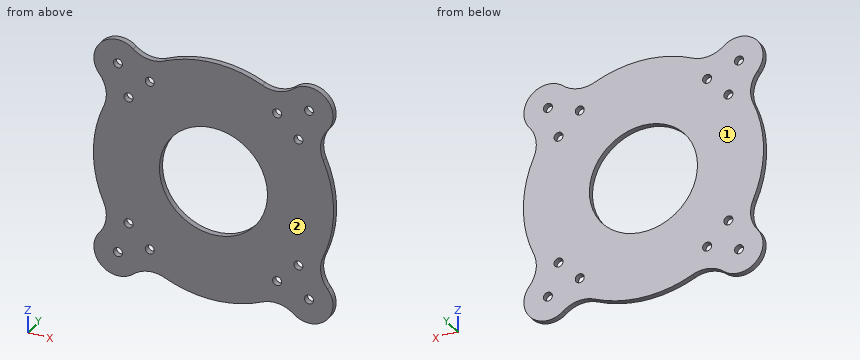
from build123d import *

# Parameters (mm, degrees)
SKETCH_1_R          = 40
SKETCH_1_R_2        = 18
EXTRUDE_1_DEPTH     = 2
EXTRUDE_2_DEPTH     = 2
FILLET_1_R          = 10
SKETCH_2_R          = 1.5
CUT_EXTRUDE_1_DEPTH = 57.603886937


with BuildPart() as part:
    # 草图1 → 凸台-拉伸1 (new body)
    with BuildSketch(Plane(origin=(0, 0, 0), x_dir=(1, 0, 0), z_dir=(0, 1, 0))):
        with Locations(Location((0, 0, 0), (0, 0, 270))):
            Circle(SKETCH_1_R)
        with Locations(Location((0, 0, 0), (0, 0, 270))):
            Circle(SKETCH_1_R_2, mode=Mode.SUBTRACT)
    extrude(amount=EXTRUDE_1_DEPTH)

    # 草图4 → 凸台-拉伸2 (add)
    with BuildSketch(Plane.XZ):
        with BuildLine():
            Line((19.091883092, 30.405591591), (26.162950904, 37.476659403))
            ThreePointArc((26.162950904, 37.476659403), (37.476659403, 37.476659403), (37.476659403, 26.162950904))
            Line((37.476659403, 26.162950904), (30.405591591, 19.091883092))
            ThreePointArc((30.405591591, 19.091883092), (19.091883092, 19.091883092), (19.091883092, 30.405591591))
        make_face()
        with BuildLine():
            Line((19.091883092, -30.405591591), (26.162950904, -37.476659403))
            ThreePointArc((26.162950904, -37.476659403), (37.476659403, -37.476659403), (37.476659403, -26.162950904))
            Line((37.476659403, -26.162950904), (30.405591591, -19.091883092))
            ThreePointArc((30.405591591, -19.091883092), (19.091883092, -19.091883092), (19.091883092, -30.405591591))
        make_face()
        with BuildLine():
            Line((-30.405591591, -19.091883092), (-37.476659403, -26.162950904))
            ThreePointArc((-37.476659403, -26.162950904), (-37.476659403, -37.476659403), (-26.162950904, -37.476659403))
            Line((-26.162950904, -37.476659403), (-19.091883092, -30.405591591))
            ThreePointArc((-19.091883092, -30.405591591), (-19.091883092, -19.091883092), (-30.405591591, -19.091883092))
        make_face()
        with BuildLine():
            Line((-19.091883092, 30.405591591), (-26.162950904, 37.476659403))
            ThreePointArc((-26.162950904, 37.476659403), (-37.476659403, 37.476659403), (-37.476659403, 26.162950904))
            Line((-37.476659403, 26.162950904), (-30.405591591, 19.091883092))
            ThreePointArc((-30.405591591, 19.091883092), (-19.091883092, 19.091883092), (-19.091883092, 30.405591591))
        make_face()
    extrude(amount=-EXTRUDE_2_DEPTH)

    # 圆角1
    fillet_1_edges = [part.edges().sort_by_distance(p)[0] for p in [
        (-22.055958672, 1, -33.369667171),
        (-33.369667171, 1, -22.055958672),
        (-33.369667171, 1, 22.055958672),
        (-22.055958672, 1, 33.369667171),
        (22.055958672, 1, 33.369667171),
        (33.369667171, 1, 22.055958672),
        (33.369667171, 1, -22.055958672),
        (22.055958672, 1, -33.369667171),
    ]]
    fillet(fillet_1_edges, radius=FILLET_1_R)

    # 草图2 → 切除-拉伸1 (cut, through all)
    with BuildSketch(Plane(origin=(0, 2, 0), x_dir=(1, 0, 0), z_dir=(0, 1, 0))):
        with Locations(Location((-21.213203436, -28.284271247, 0), (0, 0, 270))):
            Circle(SKETCH_2_R)
        with Locations(Location((-31.819805153, -31.819805153, 0), (0, 0, 270))):
            Circle(SKETCH_2_R)
        with Locations(Location((-28.284271247, -21.213203436, 0), (0, 0, 90))):
            Circle(SKETCH_2_R)
        with Locations(Location((-31.819805153, 31.819805153, 0), (0, 0, 270))):
            Circle(SKETCH_2_R)
        with Locations(Location((-21.213203436, 28.284271247, 0), (0, 0, 90))):
            Circle(SKETCH_2_R)
        with Locations(Location((-28.284271247, 21.213203436, 0), (0, 0, 270))):
            Circle(SKETCH_2_R)
        with Locations(Location((31.819805153, 31.819805153, 0), (0, 0, 270))):
            Circle(SKETCH_2_R)
        with Locations(Location((28.284271247, 21.213203436, 0), (0, 0, 90))):
            Circle(SKETCH_2_R)
        with Locations(Location((21.213203436, 28.284271247, 0), (0, 0, 270))):
            Circle(SKETCH_2_R)
        with Locations(Location((31.819805153, -31.819805153, 0), (0, 0, 270))):
            Circle(SKETCH_2_R)
        with Locations(Location((21.213203436, -28.284271247, 0), (0, 0, 90))):
            Circle(SKETCH_2_R)
        with Locations(Location((28.284271247, -21.213203436, 0), (0, 0, 270))):
            Circle(SKETCH_2_R)
    extrude(amount=-CUT_EXTRUDE_1_DEPTH, mode=Mode.SUBTRACT)


solid = part.part
Geometry: final body of the model. Coordinates: model frame, mm. Face numbers are marked on the shaded views. Give positions to 0.01 mm unless a question says otherwise; leave off trailing zeros. Order: outer loops, then holes, each group sorted by start corner. A loop starts at its lowest first (then second) coordinate and runs counter-clockwise, first axis right, second up. Notation, with made-up numbers: (-26.5, 44.25) -> (1.5, 44.25) arc R20 cw to (1.5, 50.25) -> close; hole circle Ø1 at (-11, 73). An arc over 180 degrees is marked (long way). Answer as a JSON object with one key per item and string values.
Q1. Section C-C (z = -32). Output: boundary loops of the cut face in (x, y).
Entries:
{"outline": "(-39.82, 0) -> (-33.31, 0) -> (-33.31, 2) -> (-39.82, 2) -> close; (-30.33, 0) -> (30.33, 0) -> (30.33, 2) -> (-30.33, 2) -> close; (33.31, 0) -> (39.82, 0) -> (39.82, 2) -> (33.31, 2) -> close"}
Q2. Draft query along Y for the marked faces 1 and 2. Return one class per face: released by +Y, released by -Y, zero draft, split by the parting line, or undercut.
Entries:
{"face 1": "released by +Y", "face 2": "released by -Y"}
Q3. Section B-B (x = 0). Output: boundary loops of the cut face in (y, z), plus the area to 3 significant figures.
Entries:
{"outline": "(0, -40) -> (2, -40) -> (2, -18) -> (0, -18) -> close; (0, 18) -> (2, 18) -> (2, 40) -> (0, 40) -> close", "area": "88.0 mm^2"}
Q4. Material intervals for probe 1 along Z at (x, y) = (-21, 1); probe 2 along X at (y, z) = (0.45, -31.5); probe 3 along Z at (x, y) = (30.5, 0.35), sorted ascending.
Entries:
{"probe 1": "z = -35.7 to -29.77, -26.8 to 26.8, 29.77 to 35.7", "probe 2": "x = -39.81 to -33.29, -30.35 to 30.35, 33.29 to 39.81", "probe 3": "z = -39.71 to -32.53, -31.11 to 31.11, 32.53 to 39.71"}
Q5. Section D-D (y = 1.6). State how many separate pieces and enclosed holes the cut face has, plus the area to 3 significant figures.
Entries:
{"separate pieces": "1", "enclosed holes": "13", "area": "4,740 mm^2"}
Q6. Section A-A (z = 0). Output: boundary loops of the cut face in (x, y), plus the area to 3 significant figures.
Entries:
{"outline": "(-40, 0) -> (-18, 0) -> (-18, 2) -> (-40, 2) -> close; (18, 0) -> (40, 0) -> (40, 2) -> (18, 2) -> close", "area": "88.0 mm^2"}
